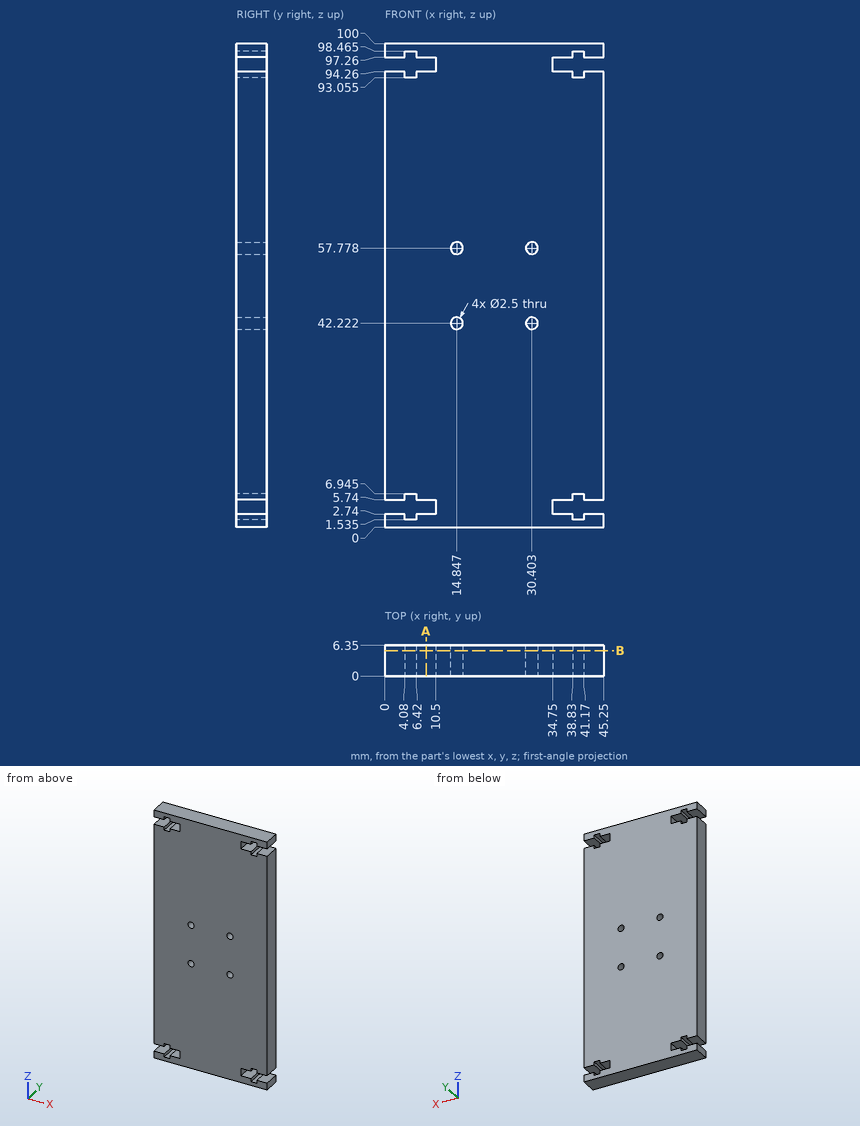
Print and shaded views of the part. All mm, measured from the part's lowest x, y and z. Coordinates: 2 decimals unless noted, no trailing zeros. Order: outer loops, then holes, each group sorted by start corner. A loop starts at its lowest first (then second) coordinate and runs counter-clockwise, first axis right, second up. Notation, with made-up numbers: (33.5, 58.5) - (55.5, 58.5) arc R22 cw to (55.5, 75.5) - close; hole circle Ø2 at (-22, 29.5). An arc over 180 degrees is marked (long way). Return JSON: item names as keys, results as strings. Group by question number.
Item 1: Pin check, flat tip, straight feed: pin 1 (0.9 mm diameter, centred on y = 4, z = 4, fed in from +X). Stop position of the tip, or through.
Item 2: Cut at B-B (y = 5.25). State how many separate pieces and enclosed holes the cut face has, plus the area to 3 significant figures.
Item 3: Drill centre lines: probe 1 along Z at (x, y) = (2, 2.75); probe 2 along Z at (x, y) = (15, 5.75). Where is each one in solid material? Low to high. Write a range as from..to.
Item 4: Cut at A-A (x = 8.5). List the corners of the cut face in (y, z), plus the area to 3 significant figures.
Check values:
{
 "1": {"pin 1": "stops at x = 34.75"},
 "2": {"separate pieces": "1", "enclosed holes": "4", "area": "4,360 mm2"},
 "3": {"probe 1": "z = 0..2.74, 5.74..94.26, 97.26..100", "probe 2": "z = 0..40.98, 43.46..56.54, 59.02..100"},
 "4": {"outline": "(0, 0) - (6.35, 0) - (6.35, 2.74) - (0, 2.74) - close; (0, 5.74) - (6.35, 5.74) - (6.35, 94.26) - (0, 94.26) - close; (0, 97.26) - (6.35, 97.26) - (6.35, 100) - (0, 100) - close", "area": "597 mm2"}
}
